Autodesk Inventor part; units mm, degrees
ref_plane "YZ Plane" through (0, 0, 0) normal (1, 0, 0) x (0, 1, 0)
ref_plane "XZ Plane" through (0, 0, 0) normal (0, 1, 0) x (-1, 0, 0)
ref_plane "XY Plane" through (0, 0, 0) normal (0, 0, 1) x (1, 0, 0)
sketch "Sketch1" plane through (0, 0, 0) normal (0, 1, 0) x (-1, 0, 0)
  line L0 (20.193, 15.748) -> (-20.193, 15.748)
  line L1 (-20.193, -15.748) -> (20.193, -15.748)
  line L2 (20.193, 15.748) -> (-20.193, -15.748) construction
  line L3 (-20.193, 15.748) -> (20.193, -15.748) construction
  line L4 (26.2784, 0) -> (13.1572, 0) construction
  line L5 (26.2784, 4.445) -> (20.193, 4.445)
  line L6 (20.193, -4.445) -> (26.2784, -4.445)
  arc A0 (26.2784, -4.445) -> (26.2784, 4.445) centre (26.2784, 0) ccw
  line L7 (0, -15.748) -> (0, 15.748) construction
  line L8 (-26.2784, 4.445) -> (-20.193, 4.445)
  line L9 (-20.193, -4.445) -> (-26.2784, -4.445)
  arc A1 (-26.2784, 4.445) -> (-26.2784, -4.445) centre (-26.2784, 0) ccw
  line L10 (20.193, -15.748) -> (20.193, -4.445)
  line L11 (20.193, 4.445) -> (20.193, 15.748)
  line L12 (-20.193, 15.748) -> (-20.193, 4.445)
  line L13 (-20.193, -4.445) -> (-20.193, -15.748)
  circle A2 centre (-26.2784, 0) radius 2.5527
  circle A3 centre (26.2784, 0) radius 2.5527
  point P0 (0, 0)
  point P1 (19.7178, 0)
  dimension "d0" = 40.386
  dimension "d1" = 31.496
  dimension "d2" = 8.89
  dimension "d5" = 5.1054
  dimension "d6" = 5.1054
extrude "Extrusion2" add sketch "Sketch1" along normal blind 6.35
sketch "Sketch5" plane through (0, 6.35, 0) normal (0, 1, 0) x (1, 0, 0)
  line L0 (-15.875, -11.43) -> (15.875, -11.43)
  line L1 (15.875, -11.43) -> (15.875, 11.43)
  line L2 (15.875, 11.43) -> (-15.875, 11.43)
  line L3 (-15.875, 11.43) -> (-15.875, -11.43)
  line L4 (-15.875, -11.43) -> (15.875, 11.43) construction
  line L5 (15.875, -11.43) -> (-15.875, 11.43) construction
  line L6 (-12.065, -7.62) -> (12.065, -7.62)
  line L7 (12.065, -7.62) -> (12.065, 7.62)
  line L8 (12.065, 7.62) -> (-12.065, 7.62)
  line L9 (-12.065, 7.62) -> (-12.065, -7.62)
  line L10 (-12.065, -7.62) -> (12.065, 7.62) construction
  line L11 (12.065, -7.62) -> (-12.065, 7.62) construction
  point P0 (0, 0)
  dimension "d17" = 31.75
  dimension "d18" = 22.86
  dimension "d19" = 3.81
  dimension "d20" = 3.81
extrude "Extrusion5" add sketch "Sketch5" along normal blind 12.446
equation "\"d0\" = 2 * imuBoxWallThickness + imuBoardLength + 2 * imuPrintError"
equation "\"d1\" = 2 * imuBoxWallThickness + imuBoardWidth + 2 * imuPrintError"
equation "\"d2\" = widthSlot"
equation "\"d7\" = imuBoxBottom"
equation "\"d17\" = imuBoxTopLength"
equation "\"d18\" = imuBoxTopWidth"
equation "\"d19\" = imuBoxWallThickness"
equation "\"d20\" = imuBoxWallThickness"
equation "\"imuBoardWidth\" = 22.86"
equation "\"imuBoardLength\" = 31.75"
equation "\"imuBoardTopThickness\" = 11.176"
equation "\"imuBoardBottomThickness\" = 5.334"
equation "\"imuBoardHoleDistance\" = 19.7104"
equation "\"imuBoxWallThickness\" = 3.81"
equation "\"widthSlot\" = 8.89"
equation "\"imuBoxBottom\" = 6.35"
equation "\"imuBoxHeight\" = 19.05"
equation "\"imuPrintError\" = 0.508"
equation "\"imuBoxTopWidth\" = imuBoardWidth"
equation "\"imuBoxTopLength\" = imuBoardLength"
properties part number "fc-GyroAccelBoxTop"
Model file for the job. Use its own axes, mm. A direction names the side the tool comes from. Coordinates: 2 decimals unless noted, no trailing zeros. Write each loop counter-clockwise with the first axis right and the second up, starting at its lowest first coordinate (ties: lowest second). Pieces come first, ordered by that corner, then holes. Notation, with made-up numbers: (6, -6) - (22, -6) arc R26 ccw to (22, 31) - close; hole circle Ø11 at (50.5, 58.25). An arc over 180 degrees is marked (long way). Use a Markdown table: item, result. Add a question column.
Item 1: Band-saw the part on D-D, the plane y = 10. Write the cut outline in (x, z) (3 decimals), and give its area (3 significant figures).
Item 2: Band-saw the part on B-B, the plane y = 5.75. Write the cut outline in (x, z) (3 decimals).
Item 3: Drill centre lines: line 1 along Z through (x, y) = (0, 9.75); line 2 along X through (y, z) = (11.5, 3) (3 decimals); line 3 along Z through (x, y) = (-13.5, 8). Where is each one in solid material? Low to high.
Item 4: Drop flat-ended pins along their axis: pin 1 (3 mm diameter, centred on x = -22, y = 1.5, fed in from +Z) (3 decimals); pin 2 (3.5 mm diameter, centred on x = 0, y = 12.5, fed in from +Z); pin 3 (3.5 mm diameter, centred on y = 12, z = 0.5, fed in from -X) (3 decimals); pin 4 (17 mm diameter, centred on x = -4, z = 2, fed in from +Y). Give the stop position or say it passes through.
Item 5: 3-axis set-ups, long thin cutter, end or side, ignore diameter. For faces 1 (the face through (20.193, 3, -10)), 2 (the face through (0, 6.35, 0)), 3 (the face through (-20.193, 3, 10)), 4 (the face through (-23, 3, -4.445)), 5 (the face through (0, 12, 11.43)): which of +Z, -Z, +X, -X, +Y, -Y reach the whole face in a straight line?
Item 6: Two-plate mould, pull along Z, no slides. Class faces 6 (the face through (20.193, 3, 10)), 7 (the face through (12.065, 12, 0)), 8 (the face through (23, 3, 4.445)): pulls with the +Z half, pulls with the -Z half, needs draft (parallel to the pull), parting line crosses it, or undercut.
Item 7: Band-saw the part on C-C, the plane x = -1.5. Write the cut outline in (y, z).
Item 8: Band-saw the part on A-A, the plane z = 0. Write the cut outline in (x, y) (3 decimals), and give its area (3 significant figures).
A:
| question | item | result |
|---|---|---|
| 1 | outline | (-15.875, -11.43) - (15.875, -11.43) - (15.875, 11.43) - (-15.875, 11.43) - close; hole (-12.065, -7.62) - (12.065, -7.62) - (12.065, 7.62) - (-12.065, 7.62) - close |
| 1 | area | 358 mm² |
| 2 | outline | (-26.278, -4.445) - (-20.193, -4.445) - (-20.193, -15.748) - (20.193, -15.748) - (20.193, -4.445) - (26.278, -4.445) arc R4.445 ccw to (26.278, 4.445) - (20.193, 4.445) - (20.193, 15.748) - (-20.193, 15.748) - (-20.193, 4.445) - (-26.278, 4.445) arc R4.445 ccw to start; hole circle Ø5.105 at (-26.278, 0); hole circle Ø5.105 at (26.278, 0) |
| 3 | line 1 | z = -11.43 to -7.62, 7.62 to 11.43 |
| 3 | line 2 | x = -15.875 to -12.065, 12.065 to 15.875 |
| 3 | line 3 | z = -11.43 to 11.43 |
| 4 | pin 1 | stops at z = 4.445 |
| 4 | pin 2 | stops at z = 11.43 |
| 4 | pin 3 | stops at x = -15.875 |
| 4 | pin 4 | stops at y = 18.8 |
| 5 | face 1 | -Z, +X, +Y, -Y |
| 5 | face 2 | +Y |
| 5 | face 3 | +Z, -X, +Y, -Y |
| 5 | face 4 | -Z, -X, +Y, -Y |
| 5 | face 5 | +Z, +X, -X, +Y |
| 6 | face 6 | needs draft |
| 6 | face 7 | undercut |
| 6 | face 8 | pulls with the +Z half |
| 7 | outline | (0, -15.75) - (6.35, -15.75) - (6.35, -11.43) - (18.8, -11.43) - (18.8, -7.62) - (6.35, -7.62) - (6.35, 7.62) - (18.8, 7.62) - (18.8, 11.43) - (6.35, 11.43) - (6.35, 15.75) - (0, 15.75) - close |
| 8 | outline | (-30.723, 0) - (-28.831, 0) - (-28.831, 6.35) - (-30.723, 6.35) - close; (-23.726, 0) - (23.726, 0) - (23.726, 6.35) - (15.875, 6.35) - (15.875, 18.796) - (12.065, 18.796) - (12.065, 6.35) - (-12.065, 6.35) - (-12.065, 18.796) - (-15.875, 18.796) - (-15.875, 6.35) - (-23.726, 6.35) - close; (28.831, 0) - (30.723, 0) - (30.723, 6.35) - (28.831, 6.35) - close |
| 8 | area | 420 mm² |
